Could you check a few things on this model? Use its own coordinates, in mm. A direction names the side the tool comes from. Give positions to 0.01 mm unless a question says otherwise; leave off trailing zeros. Write each loop counter-clockwise with the first axis right and the second up, starting at its lowest first coordinate (ties: lowest second). Pieces come first, ordered by that corner, then holes. Notation, with made-up numbers: (-35, 30.25) - (-22, 30.25) arc R10 ccw to (-22, 38.25) - close; hole circle Ø7 at (-10, -39). An arc over 180 degrees is marked (long way). Use one line per item in the form item = value.
Autodesk Fusion 360 part; units mm, degrees
sketch "Sketch1" plane through (0, 0, 0) normal (0, 0, 1) x (1, 0, 0)
  line L0 (21.6826, 76.2435) -> (61.6826, 76.2435)
  line L1 (61.6826, 76.2435) -> (61.6826, 61.2435)
  line L2 (21.6826, 76.2435) -> (21.6826, 61.2435)
  line L3 (61.6826, 61.2435) -> (64.1826, 61.2435)
  line L4 (21.6826, 61.2435) -> (19.1826, 61.2435)
  line L5 (64.1826, 61.2435) -> (64.1826, 51.2435)
  line L6 (19.1826, 61.2435) -> (19.1826, 51.2435)
  line L7 (64.1826, 51.2435) -> (61.6826, 51.2435)
  line L8 (19.1826, 51.2435) -> (21.6826, 51.2435)
  line L9 (21.6826, 51.2435) -> (21.6826, 36.2435)
  line L10 (61.6826, 51.2435) -> (61.6826, 36.2435)
  line L11 (61.6826, 36.2435) -> (21.6826, 36.2435)
  circle A0 centre (41.6826, 56.2435) radius 7.5
  dimension "d1" = 40
  dimension "d2" = 15
  dimension "d3" = 15
  dimension "d4" = 2.5
  dimension "d5" = 2.5
  dimension "d6" = 10
  dimension "d7" = 10
  dimension "d8" = 2.5
  dimension "d9" = 2.5
  dimension "d10" = 15
  dimension "d11" = 15
  dimension "d12" = 15
  dimension "d13" = 20
  dimension "d14" = 22.5
extrude "Extrude1" add sketch "Sketch1" along normal blind 2.5
1. For pin 1 (1.2 mm diameter, centred on x = 63, z = 1, fed in from -Y); pin 2 (0.8 mm diameter, centred on y = 43.5, z = 1.5, fed in from +X); pin 3 (0.8 mm diameter, centred on x = 21, z = 1, fed in from +Y); pin 4 (9 mm diameter, centred on x = 41.68, y = 56.24, fed in from -Z), each with a flat end and sliding along its axis, tell me the tip position at first contact or that it passes through.
Response values:
pin_1 = 51.24
pin_2 = 61.68
pin_3 = 61.24
pin_4 = through
2. Imagine slicing it at C-C, the plane y = 55. List the corners of the cut face in (x, z) for me.
Response values:
outline = (19.18, 0) - (34.29, 0) - (34.29, 2.5) - (19.18, 2.5) - close; (49.08, 0) - (64.18, 0) - (64.18, 2.5) - (49.08, 2.5) - close
3. If we mould it in two halves opening along X, with no side actions, what happens to faces 1 (the face through (45.14, 62.9, 1.23)), 2 (the face through (19.183, 56, 1)), 3 (the face through (20, 51.244, 1))? For each: pulls with the +X half, pulls with the -X half, needs draft (parallel to the pull), parting line crosses it, or undercut.
Response values:
face_1 = undercut
face_2 = pulls with the -X half
face_3 = needs draft
4. Which directions (+Z, -Z, +X, -X, +Y, -Y) give clear straight access to the entire face, cutting with the end or side of a thin tool? Please do faces 4 (the face through (21.683, 44, 1)), 5 (the face through (20, 61.244, 1)), 6 (the face through (63, 51.244, 1)), 7 (the face through (51, 57, 2.5)), 8 (the face through (63, 61.244, 1)).
Response values:
face_4 = +Z, -Z, -X, -Y
face_5 = +Z, -Z, -X, +Y
face_6 = +Z, -Z, +X, -Y
face_7 = +Z, +X, -X, +Y, -Y
face_8 = +Z, -Z, +X, +Y
5. Imagine slicing it at B-B, the plane z = 1.15. List the corners of the cut face in (x, y) for me, and give its area (3 significant figures).
Response values:
outline = (19.18, 51.24) - (21.68, 51.24) - (21.68, 36.24) - (61.68, 36.24) - (61.68, 51.24) - (64.18, 51.24) - (64.18, 61.24) - (61.68, 61.24) - (61.68, 76.24) - (21.68, 76.24) - (21.68, 61.24) - (19.18, 61.24) - close; hole circle Ø15 at (41.68, 56.24)
area = 1,470 mm²
6. If I drill on line 1 (Y direction, x = 43.5, z = 0.6); line 2 (X direction, y = 41, z = 1.2); line 3 (X direction, y = 53, z = 2.1), over which ranges is the centre line in solid material (lowest first)? Write a range as from..to.
Response values:
line_1 = 36.24..48.97, 63.52..76.24
line_2 = 21.68..61.68
line_3 = 19.18..34.92, 48.44..64.18
7. Imagine slicing it at D-D, the plane y = 66.5. List the corners of the cut face in (x, z) for me, and give its area (3 significant figures).
Response values:
outline = (21.68, 0) - (61.68, 0) - (61.68, 2.5) - (21.68, 2.5) - close
area = 100 mm²
8. Imagine slicing it at A-A, the plane x = 40. List the corners of the cut face in (y, z) for me, and give its area (3 significant figures).
Response values:
outline = (36.24, 0) - (48.93, 0) - (48.93, 2.5) - (36.24, 2.5) - close; (63.55, 0) - (76.24, 0) - (76.24, 2.5) - (63.55, 2.5) - close
area = 63.5 mm²
